from build123d import *

# Parameters (mm, degrees)
SKETCH_W        = 144
SKETCH_H        = 80
PAD_DEPTH       = 5
FILLET_R        = 4
SKETCH001_R     = 2.25
POCKET_DEPTH    = 10
SKETCH002_R     = 3.75
POCKET001_DEPTH = 3
SKETCH003_W     = 40
SKETCH003_H     = 40
POCKET002_DEPTH = 5
SKETCH004_W     = 8
SKETCH004_H     = 8
PAD001_DEPTH    = 5
SKETCH005_R     = 1.75
POCKET003_DEPTH = 5
FILLET001_R     = 2
SKETCH006_R     = 3
POCKET004_DEPTH = 2


with BuildPart() as part:
    # Sketch → Pad (new body)
    with BuildSketch(Plane.XY):
        with Locations((72, 40)):
            Rectangle(SKETCH_W, SKETCH_H)
    extrude(amount=PAD_DEPTH)

    # Fillet
    fillet_edges = [part.edges().sort_by_distance(p)[0] for p in [
        (144, 0, 2.5),
        (144, 80, 2.5),
        (0, 0, 2.5),
        (0, 80, 2.5),
    ]]
    fillet(fillet_edges, radius=FILLET_R)

    # Sketch001 (on Face5 of Fillet) → Pocket (cut)
    with BuildSketch(Plane.XY.offset(5)):
        with Locations((72, 9)):
            Circle(SKETCH001_R)
        with Locations((72, 71)):
            Circle(SKETCH001_R)
    extrude(amount=-POCKET_DEPTH, mode=Mode.SUBTRACT)

    # Sketch002 (on Face5 of Pocket) → Pocket001 (cut)
    with BuildSketch(Plane.XY.offset(5)):
        with Locations((72, 9)):
            Circle(SKETCH002_R)
        with Locations((72, 71)):
            Circle(SKETCH002_R)
    extrude(amount=-POCKET001_DEPTH, mode=Mode.SUBTRACT)

    # Sketch003 (on Face5 of Pocket001) → Pocket002 (cut)
    with BuildSketch(Plane.XY.offset(5)):
        with Locations((72, 40)):
            Rectangle(SKETCH003_W, SKETCH003_H)
    extrude(amount=-POCKET002_DEPTH, mode=Mode.SUBTRACT)

    # Sketch004 (on Face5 of Pocket002) → Pad001 (join)
    with BuildSketch(Plane.XY.offset(5)):
        with Locations((56, 56)):
            Rectangle(SKETCH004_W, SKETCH004_H)
        with Locations((56, 24)):
            Rectangle(SKETCH004_W, SKETCH004_H)
        with Locations((88, 24)):
            Rectangle(SKETCH004_W, SKETCH004_H)
        with Locations((88, 56)):
            Rectangle(SKETCH004_W, SKETCH004_H)
    extrude(amount=-PAD001_DEPTH)

    # Sketch005 (on Face28 of Pad001) → Pocket003 (cut)
    with BuildSketch(Plane.XY.offset(5)):
        with Locations((56, 56)):
            Circle(SKETCH005_R)
        with Locations((88, 56)):
            Circle(SKETCH005_R)
        with Locations((56, 24)):
            Circle(SKETCH005_R)
        with Locations((88, 24)):
            Circle(SKETCH005_R)
    extrude(amount=-POCKET003_DEPTH, mode=Mode.SUBTRACT)

    # Fillet001
    fillet001_edges = [part.edges().sort_by_distance(p)[0] for p in [
        (60, 52, 2.5),
        (60, 60, 2.5),
        (52, 52, 2.5),
        (52, 28, 2.5),
        (60, 28, 2.5),
        (60, 20, 2.5),
        (84, 28, 2.5),
        (92, 28, 2.5),
        (84, 20, 2.5),
        (84, 60, 2.5),
        (84, 52, 2.5),
        (92, 52, 2.5),
    ]]
    fillet(fillet001_edges, radius=FILLET001_R)

    # Sketch006 (on Face40 of Fillet001) → Pocket004 (cut)
    with BuildSketch(Plane.XY.offset(5)):
        with Locations((56, 24)):
            Circle(SKETCH006_R)
        with Locations((56, 56)):
            Circle(SKETCH006_R)
        with Locations((88, 56)):
            Circle(SKETCH006_R)
        with Locations((88, 24)):
            Circle(SKETCH006_R)
    extrude(amount=-POCKET004_DEPTH, mode=Mode.SUBTRACT)


solid = part.part
Build history of the part. All positions in model axes, mm. A direction names the side the tool comes from. Give positions to 0.01 mm unless a question says otherwise; leave off trailing zeros. Order: outer loops, then holes, each group sorted by start corner. A loop starts at its lowest first (then second) coordinate and runs counter-clockwise, first axis right, second up. Notation, with made-up numbers: M 88.25,0.5 L 117.25,0.5 A15 cw 117.25,21.5 Z; hole C -4.5,64 d8. An arc over 180 degrees is marked long. Use one line per item in the form item = value.
Q1. Slice it at D-D, the plane z = 1.15. State how many separate pieces and enclosed holes the cut face has, and give its area (3 significant figures).
Conclusion:
separate_pieces = 1
enclosed_holes = 7
area = 10,100 mm2
Q2. Pull direction X, two halves, no side cores. Call faces 4 (the cylindrical face through (1.141, 1.203, 2.535)), 5 (the flat face through (84, 24, 3)), 6 (the flat face through (87, 58, 0)), 7 (the flat face through (144, 39, 2)): released by +X, released by -X, zero draft, split by the parting line, or undercut.
Conclusion:
face_4 = released by -X
face_5 = undercut
face_6 = zero draft
face_7 = released by +X
Q3. Wall check: probe 1 along Y at (x, z) = (56, 4.2); probe 2 along Y at (x, z) = (88, 0.8); probe 3 along X at (y, z) = (36, 0.6). Give the ranges that are in metal, low to high.
Conclusion:
probe_1 = 0 to 21, 27 to 28, 52 to 53, 59 to 80
probe_2 = 0 to 22.25, 25.75 to 28, 52 to 54.25, 57.75 to 80
probe_3 = 0 to 52, 92 to 144
Q4. Which spindle directions (+Z, -Z, +X, -X, +Y, -Y) get a long thin tool onto all of the face, cutting with end or side? Do faces 1 (the flat face through (0, 39, 2)), 2 (the flat face through (60, 56, 3)), 3 (the flat face through (58, 24, 3)). Say none if no direction does.
Conclusion:
face_1 = +Z, -Z, -X, +Y, -Y
face_2 = +Z, -Z
face_3 = +Z
Q5. Slice it at A-A, the plane y = 46. Write the cut outline in (x, z).
Conclusion:
outline = M 0,0 L 52,0 L 52,5 L 0,5 Z; M 92,0 L 144,0 L 144,5 L 92,5 Z
Q6. Slice it at C-C, the plane x = 88. Write the cut outline in (y, z), and give its area (3 significant figures).
Conclusion:
outline = M 0,0 L 22.25,0 L 22.25,3 L 21,3 L 21,5 L 0,5 Z; M 25.75,0 L 28,0 L 28,5 L 27,5 L 27,3 L 25.75,3 Z; M 52,0 L 54.25,0 L 54.25,3 L 53,3 L 53,5 L 52,5 Z; M 57.75,0 L 80,0 L 80,5 L 59,5 L 59,3 L 57.75,3 Z
area = 235 mm2
Q7. Slice it at B-B, the plane y = 56. Write the cut outline in (x, z), and give its area (3 significant figures).
Conclusion:
outline = M 0,0 L 54.25,0 L 54.25,3 L 53,3 L 53,5 L 0,5 Z; M 57.75,0 L 60,0 L 60,5 L 59,5 L 59,3 L 57.75,3 Z; M 84,0 L 86.25,0 L 86.25,3 L 85,3 L 85,5 L 84,5 Z; M 89.75,0 L 144,0 L 144,5 L 91,5 L 91,3 L 89.75,3 Z
area = 555 mm2
Q8. Pin check, flat tips, straight feed: P1, Ø7, axis at x = 72, y = 71, coming from the +Z side; P2, Ø4, axis at x = 88, y = 56, coming from the +Z side. Stop position of each tip, or through.
Conclusion:
P1 = 2
P2 = 3
